Can you work these out from the model? Positions are in its coordinate system, mm. A direction names the side the tool comes from. Round coordinates to 2 decimals unless told otherwise and drop trailing zeros. Order: outer loops, then holes, each group sorted by start corner. A loop starts at its lowest first (then second) coordinate and runs counter-clockwise, first axis right, second up. Notation, with made-up numbers: M 57,70.5 L 72,70.5 A17 cw 72,79.5 Z; hole C 30.5,-27 d10. An arc over 180 degrees is marked long. One line per question, with ' | ' between items.
```python
from build123d import *

# Parameters (mm, degrees)
SKETCH2_W         = 6
SKETCH2_H         = 1
SLOT_DEPTH        = 1.5
CIRPATTERN1_COUNT = 2
CIRPATTERN1_ANGLE = 90


with BuildPart() as part:
    # BodySke → Base-Revolve (revolve)
    with BuildSketch(Plane.XY, mode=Mode.PRIVATE) as base_revolve_sk:
        with BuildLine():
            Line((0, 0), (30.016891186, 0))
            Line((30.016891186, 0), (30.016891186, 2))
            Line((30.016891186, 2), (3.470777776, 2))
            Line((3.470777776, 2), (3.470777776, 4.052285877))
            Line((3.470777776, 4.052285877), (1.246697171, 4.052285877))
            ThreePointArc((1.246697171, 4.052285877), (0.326924477, 2.117338651), (0, 0))
        make_face()
    revolve(base_revolve_sk.sketch.rotate(Axis((-15.875, 0, 0), (1, 0, 0)), 90), axis=Axis((-15.875, 0, 0), (1, 0, 0)))

    # Sketch2 → Slot (cut)
    with BuildSketch(Plane(origin=(0, 0, 0), x_dir=(0, 0, -1), z_dir=(1, 0, 0))):
        Rectangle(SKETCH2_W, SKETCH2_H)
    extrude(amount=SLOT_DEPTH, mode=Mode.SUBTRACT)

    # Sketch3 → Cross section 0
    with BuildSketch(Plane(origin=(0, 0, 0), x_dir=(0, 0, -1), z_dir=(1, 0, 0))):
        with BuildLine():
            Line((0.415, -1.72), (-0.415, -1.72))
            Line((-0.415, -1.72), (-0.415, 1.72))
            Line((-0.415, 1.72), (0.415, 1.72))
            Line((0.415, 1.72), (0.415, -1.72))
        make_face()
    # Sketch4 → Cross section 1
    with BuildSketch(Plane(origin=(2.33, 0, 0), x_dir=(0, 0, -1), z_dir=(1, 0, 0))):
        with BuildLine():
            Line((0.2075, -0.2075), (-0.2075, -0.2075))
            Line((-0.2075, -0.2075), (-0.2075, 0.2075))
            Line((-0.2075, 0.2075), (0.2075, 0.2075))
            Line((0.2075, 0.2075), (0.2075, -0.2075))
        make_face()
    cross = loft(mode=Mode.SUBTRACT)

    # CirPattern1: Cross ×2 about axis
    cirpattern1_axis = Axis((0, 0, 0), (1, 0, 0))
    for i in range(1, CIRPATTERN1_COUNT):
        add(cross.rotate(cirpattern1_axis, i * CIRPATTERN1_ANGLE / (CIRPATTERN1_COUNT - 1)), mode=Mode.SUBTRACT)


solid = part.part
```
(1) If we section it at A-A on x = 12.25: Please give me the cut outline in (y, z), plus the area to 3 significant figures.
Final values:
outline: C 0,0 d4 | area: 12.6 mm^2
(2) Will these pins go through, and if not, where does the flat tip stop? pin 1 Ø0.7 at (x, z) = (0.5, -2) entering from +Y; pin 2 Ø0.5 at (y, z) = (0, -2) entering from -X; pin 3 Ø0.7 at (x, z) = (1, -2) entering from -Y.
Final values:
pin 1: y = 2.77 | pin 2: x = 1.5 | pin 3: y = -3.65
(3) Please list where these lines run through material, in increasing order: probe 1 along X at (y, z) = (1.5, -1.25); probe 2 along Z at (x, y) = (21.5, 0.25); probe 3 along Z at (x, y) = (11.5, -1). Write a range as [from, to].
Final values:
probe 1: [0.28, 30.02] | probe 2: [-1.98, 1.98] | probe 3: [-1.73, 1.73]
(4) On a 3-axis mill with a long thin cutter (end or side, diameter ignored), from which of +Z, -Z, +X, -X, +Y, -Y can I reach the whole of each face in a straight line? I mean faces 1 (the flat face through (1.5, 0, -2)), 2 (the cylindrical face through (17, 2, 0)). Say none if no direction works.
Final values:
face 1: -X | face 2: +X
(5) Thinking about a two-plate mould opening in Y: for faces 3 (the cylindrical face through (2.343, -1.217, 3.865)), 4 (the flat face through (1, -0.5, -2)), 5 (the flat face through (30.017, 0, 0)), which applies, released by +Y, released by -Y, zero draft, split by the parting line, or undercut?
Final values:
face 3: split by the parting line | face 4: undercut | face 5: zero draft
